Build history of the part. All positions in model axes, mm. A direction names the side the tool comes from. Round coordinates to 2 decimals unless told otherwise and drop trailing zeros. Loops run counter-clockwise (first coordinate to the right, second up) from the corner with the lowest first, then second, coordinate; pieces in that order, holes last. Notation, with made-up numbers: (27, -5.5) - (40, -5.5) arc R20 cw to (40, 23.5) - close; hole circle Ø2 at (58.25, 28). An arc over 180 degrees is marked (long way). Put each result on its own line as item: value. Start each with the question number.
from build123d import *

# Parameters (mm, degrees)
BOSS_EXTRUDE1_DEPTH = 19.05
SKETCH2_R           = 22.5
CUT_EXTRUDE1_DEPTH  = 17.05
FILLET1_R           = 2
FILLET2_R           = 1


with BuildPart() as part:
    # Sketch1 → Boss-Extrude1 (new body)
    with BuildSketch(Plane(origin=(0, 0, 0), x_dir=(1, 0, 0), z_dir=(0, 1, 0))):
        with BuildLine():
            Line((30.602986827, -26.563786798), (41.395992873, -26.563786798))
            ThreePointArc((41.395992873, -26.563786798), (41.999506373, -26.313803321), (42.24948985, -25.710289821))
            Line((42.24948985, -25.710289821), (42.24948985, 54.289710179))
            Line((42.24948985, 54.289710179), (42.24948985, 61.876099251))
            ThreePointArc((42.24948985, 61.876099251), (41.999506373, 62.479612751), (41.395992873, 62.729596228))
            Line((41.395992873, 62.729596228), (-33.347013177, 62.729596228))
            ThreePointArc((-33.347013177, 62.729596228), (-33.950526677, 62.479612751), (-34.200510153, 61.876099251))
            Line((-34.200510153, 61.876099251), (-34.200510153, 49.376099251))
            ThreePointArc((-34.200510153, 49.376099251), (-33.950526677, 48.772585752), (-33.347013177, 48.522602275))
            Line((-33.347013177, 48.522602275), (28.895992873, 48.522602275))
            ThreePointArc((28.895992873, 48.522602275), (29.499506373, 48.272618798), (29.74948985, 47.669105298))
            Line((29.74948985, 47.669105298), (29.74948985, 30.255903719))
            ThreePointArc((29.74948985, 30.255903719), (29.176620882, 29.44986091), (28.227035694, 29.725853361))
            ThreePointArc((28.227035694, 29.725853361), (-34.205400414, 7.989675013), (28.227035694, -13.746503336))
            ThreePointArc((28.227035694, -13.746503336), (29.176620882, -13.470510884), (29.74948985, -14.276553693))
            Line((29.74948985, -14.276553693), (29.74948985, -25.710289821))
            ThreePointArc((29.74948985, -25.710289821), (29.999473327, -26.313803321), (30.602986827, -26.563786798))
        make_face()
    extrude(amount=BOSS_EXTRUDE1_DEPTH)

    # Sketch2 → Cut-Extrude1 (cut)
    with BuildSketch(Plane(origin=(0, 19.05, 0), x_dir=(1, 0, 0), z_dir=(0, 1, 0))):
        with BuildLine():
            Line((39.74948985, -24.063786798), (39.74948985, 60.229596228))
            Line((39.74948985, 60.229596228), (-31.700510153, 60.229596228))
            Line((-31.700510153, 60.229596228), (-31.700510153, 51.022602275))
            Line((-31.700510153, 51.022602275), (28.895992873, 51.022602275))
            ThreePointArc((28.895992873, 51.022602275), (31.267273326, 50.040385751), (32.24948985, 47.669105298))
            Line((32.24948985, 47.669105298), (32.24948985, 30.255903719))
            ThreePointArc((32.24948985, 30.255903719), (29.998615619, 27.088860136), (26.267575972, 28.173269194))
            ThreePointArc((26.267575972, 28.173269194), (-31.705400414, 7.989675013), (26.267575972, -12.193919168))
            ThreePointArc((26.267575972, -12.193919168), (29.998615619, -11.109510111), (32.24948985, -14.276553693))
            Line((32.24948985, -14.276553693), (32.24948985, -24.063786798))
            Line((32.24948985, -24.063786798), (39.74948985, -24.063786798))
        make_face()
        with Locations(Location((0.794599586, 7.989675013, 0), (0, 0, 270))):
            Circle(SKETCH2_R, mode=Mode.SUBTRACT)
    extrude(amount=-CUT_EXTRUDE1_DEPTH, mode=Mode.SUBTRACT)

    # Fillet1
    fillet1_edges = [part.edges().sort_by_distance(p)[0] for p in [
        (39.74948985, 10.525, 24.063786798),
        (32.24948985, 10.525, 24.063786798),
        (-31.700510153, 10.525, -51.022602275),
        (-31.700510153, 10.525, -60.229596228),
        (39.74948985, 10.525, -60.229596228),
    ]]
    fillet(fillet1_edges, radius=FILLET1_R)

    # Fillet2
    fillet2_edges = [part.edges().sort_by_distance(p)[0] for p in [
        (32.24948985, 2, 18.170170245),
        (29.998615619, 2, 11.109510111),
        (-31.705400414, 2, -7.989675013),
        (29.998615619, 2, -27.088860136),
        (32.24948985, 2, -38.962504508),
        (31.267273326, 2, -50.040385751),
        (35.99948985, 2, 24.063786798),
        (39.74948985, 2, -18.082904715),
        (4.024489848, 2, -60.229596228),
        (-31.700510153, 2, -55.626099251),
        (-0.40225864, 2, -51.022602275),
        (39.163703412, 2, -59.64380979),
        (-31.114723716, 2, -59.64380979),
        (-31.114723716, 2, -51.608388712),
        (39.163703412, 2, 23.47800036),
        (32.835276288, 2, 23.47800036),
    ]]
    fillet(fillet2_edges, radius=FILLET2_R)


solid = part.part
Item 1: Drill centre lines: probe 1 along Z at (x, y) = (-28, 14.75); probe 2 along X at (y, z) = (10.5, -31); probe 3 along X at (y, z) = (17.5, -34). Where is each one in solid material? Low to high. Write a range as [from, to].
Item 2: Slice it at A-A (y = 8.25). Give the number of separate pieces and of enclosed holes in the cut face, plus the area to 3 significant figures.
Item 3: Slice it at B-B (x = 36.5). Give the cut face in (y, z), plus the area to 3 significant figures.
Item 4: Two-plate mould, pull along Z, no slides. Class faces 4 (the flat face through (5, 9, -62.73)), 5 (the flat face through (36, 11, 24.064)), 6 (the flat face through (42.249, 9, -17)): pulls with the +Z half, pulls with the -Z half, needs draft (parallel to the pull), parting line crosses it, or undercut.
Item 5: Drop flat-ended pins along their axis: pin 1 Ø3 at (x, z) = (33, -7) entering from +Y; pin 2 Ø5.5 at (x, y) = (37.5, 13.5) entering from +Z; pin 3 Ø10 at (y, z) = (13.5, 8) entering from -X. Give the stop position or say it passes through.
Item 6: Which spindle directions (+Z, -Z, +X, -X, +Y, -Y) get a long thin tool onto all of the face, cutting with end or side? Do faces 1 (the flat face through (24, 19.05, -31)), 2 (the cylindrical face through (31.24, 11.14, -50.07)), 3 (the flat face through (29.749, 9, 20)). Say none if no direction does.
Computed values:
1. probe 1: z = [-62.73, -60.23], [-51.02, -48.52], [-27.89, -23.06], [7.08, 11.91]
1. probe 2: x = [-25.58, -22.16], [23.75, 27.17], [29.75, 32.25], [39.75, 42.25]
1. probe 3: x = [-22.62, -18.69], [20.28, 24.21], [29.75, 32.25], [39.75, 42.25]
2. separate pieces: 2
2. enclosed holes: 1
2. area: 2,730 mm^2
3. outline: (0, -62.73) - (19.05, -62.73) - (19.05, -60.23) - (3, -60.23) arc R1 cw to (2, -59.23) - (2, 23.06) arc R1 cw to (3, 24.06) - (19.05, 24.06) - (19.05, 26.56) - (0, 26.56) - close
3. area: 264 mm^2
4. face 4: pulls with the -Z half
4. face 5: undercut
4. face 6: needs draft
5. pin 1: stops at y = 2
5. pin 2: stops at z = 26.56
5. pin 3: stops at x = -32.44
6. face 1: +Z, -Z, +X, -X, +Y
6. face 2: +Y
6. face 3: +Z, +Y, -Y
